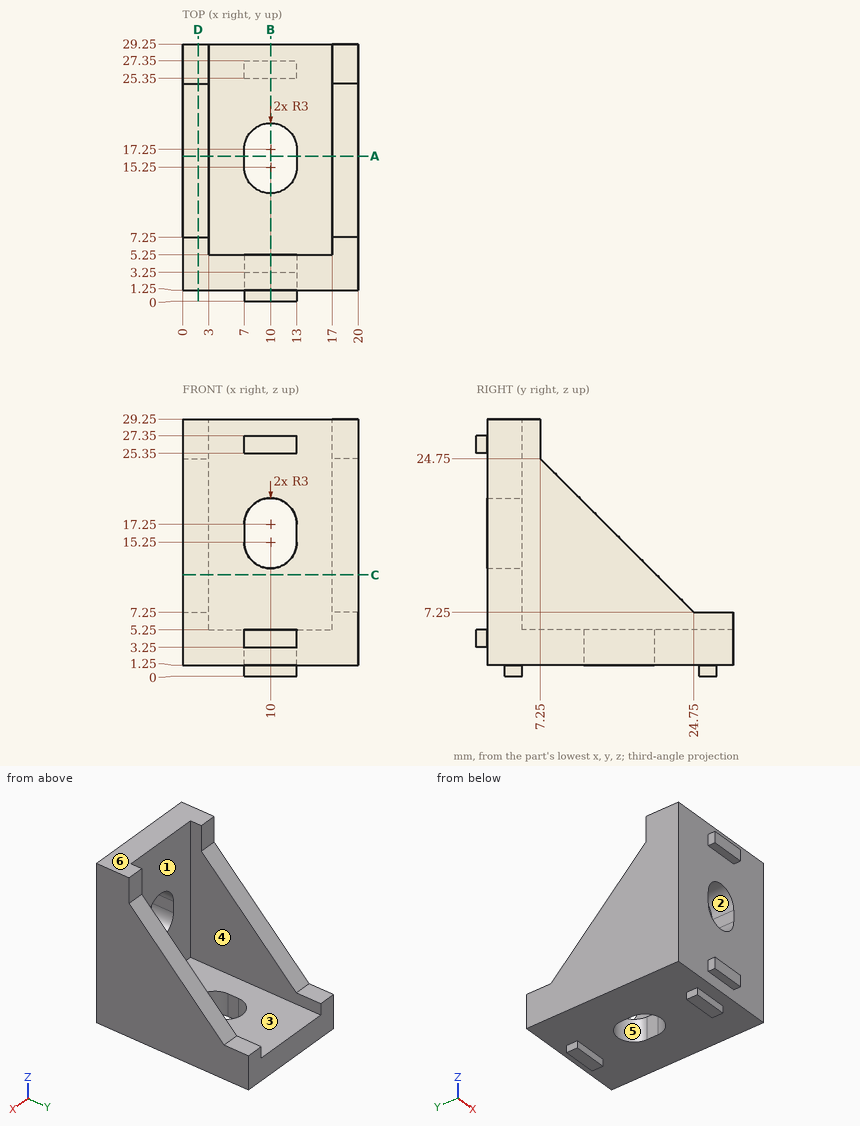
For this review, use the dimensioned drawing (mm, ordinates from the lowest corner) and the shaded views. A direction names the side the tool comes from. Coordinates: 2 decimals unless noted, no trailing zeros. Loops run counter-clockwise (first coordinate to the right, second up) from the corner with the lowest first, then second, coordinate; pieces in that order, holes last. Notation, with made-up numbers: (35, -5) -> (83, -5) arc R18 cw to (83, 25) -> close; hole circle Ø7 at (-28, 79). An arc over 180 degrees is marked (long way). Return JSON: item names as keys, results as strings. Group by question number.
(1) To check wall thickness, follow L1, parallel to X at y = 23, z = 8.75; L2, parallel to Z at x = 13, y = 24.5. State the ranges of each line that lie inside material, in increasing order.
(2) Consider section A-A, the plane y = 16.5. Give the boundary of the cut face in (x, z), plus the area to 4 significant figures.
(3) Consider section D-D, the plane x = 1.75. Give the boundary of the cut face in (y, z), plus the area to 3 significant figures.
(4) Mouldability with a two-part tool opening along Z and no side actions: class the marked faces 1, 2 and 3 as pulls with the +Z half, pulls with the -Z half, needs draft (parallel to the pull), parting line crosses it, or undercut.
(5) For pin 1 Ø0.6 at (y, z) = (26.5, 0.5) entering from -X; pin 2 Ø2 at (x, z) = (14, 21) entering from +Y; pin 3 Ø4 at (x, z) = (15.5, 10) entering from -Y, all flat-tipped, find the tip position at first contact; note any pin that passes through.
(6) Consider section C-C, the plane z = 11.5. Give the boundary of the cut face in (x, y), plus the area to 4 significant figures.
(7) Consider section B-B, the plane x = 10. Count the separate pieces of the cut face and the enclosed holes in it, plus the area to 3 significant figures.
(8) Tool access review of the marked faces 4, 5 and 6: name each direction out of +Z, -Z, +X, -X, +Y, -Y from which nothing blocks a thin tool from reaching the whole face with its end or side.
Results below:
{
 "1": {"L1": "x = 0 to 3, 17 to 20", "L2": "z = 1.25 to 5.25"},
 "2": {"outline": "(0, 1.25) -> (7, 1.25) -> (7, 5.25) -> (3, 5.25) -> (3, 15.5) -> (0, 15.5) -> close; (13, 1.25) -> (20, 1.25) -> (20, 15.5) -> (17, 15.5) -> (17, 5.25) -> (13, 5.25) -> close", "area": "117.5 mm2"},
 "3": {"outline": "(1.25, 1.25) -> (29.25, 1.25) -> (29.25, 7.25) -> (24.75, 7.25) -> (7.25, 24.75) -> (7.25, 29.25) -> (1.25, 29.25) -> close", "area": "453 mm2"},
 "4": {"face 1": "needs draft", "face 2": "undercut", "face 3": "pulls with the +Z half"},
 "5": {"pin 1": "stops at x = 7", "pin 2": "stops at y = 5.25", "pin 3": "stops at y = 1.25"},
 "6": {"outline": "(0, 1.25) -> (20, 1.25) -> (20, 20.5) -> (17, 20.5) -> (17, 5.25) -> (3, 5.25) -> (3, 20.5) -> (0, 20.5) -> close", "area": "171.5 mm2"},
 "7": {"separate pieces": "3", "enclosed holes": "0", "area": "154 mm2"},
 "8": {"face 4": "+Z, +Y", "face 5": "+Z, -Z", "face 6": "+Z, +X, -X, +Y, -Y"}
}
